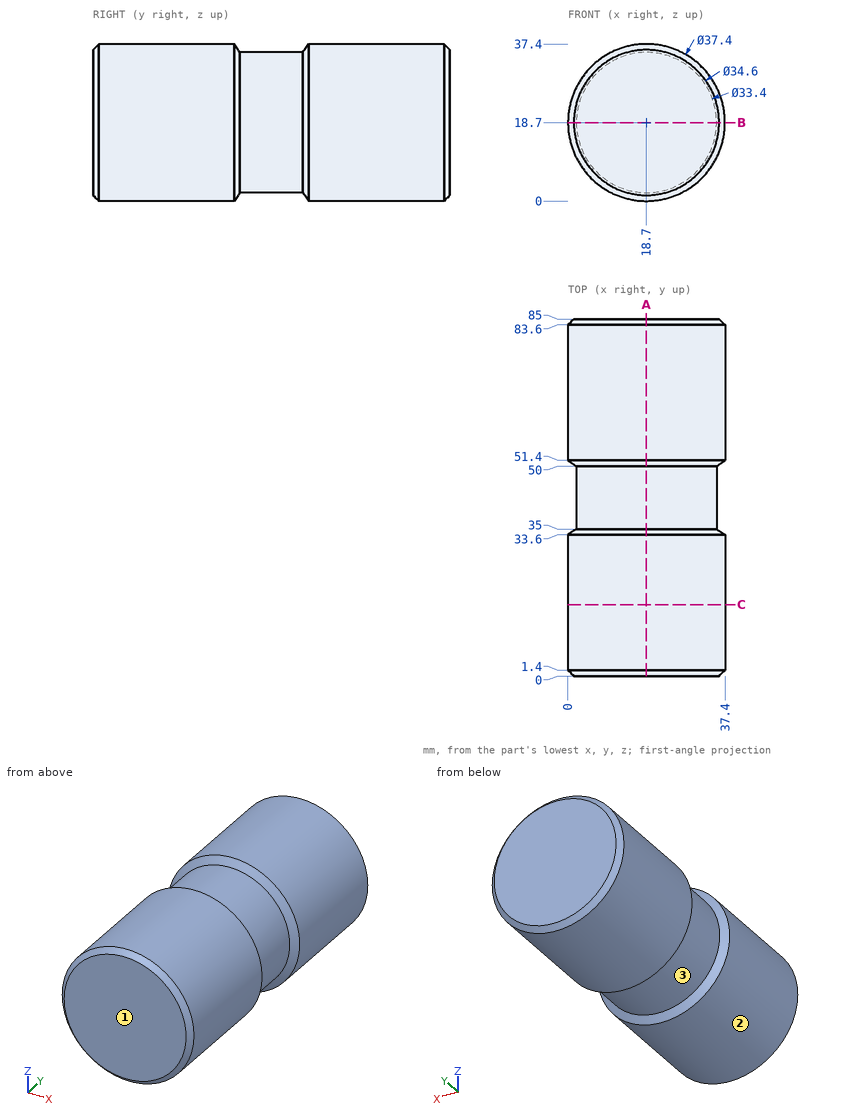
Study the drawing (mm; zero at the part's minimum x, y, z) and answer. Coordinates: 2 decimals unless noted, no trailing zeros. Write each loop counter-clockwise with the first axis right and the second up, starting at its lowest first coordinate (ties: lowest second). Pieces come first, ordered by that corner, then holes. Notation, with made-up numbers: (-21, 32) - (23, 32) arc R12 ccw to (23, 37) - close; hole circle Ø11 at (54.5, -23.5). An arc over 180 degrees is marked (long way). One line per question, with ' | ' between items.
1) Consider probe 1 along Z at (x, y) = (19.5, 78.5); probe 2 along Y at (x, z) = (2, 26) (1 decimal); probe 3 along X at (y, z) = (47.5, 19). Determine where each line is inside the solid, lowest interval first. Write a range as [from, to].
Checks:
probe 1: [0.02, 37.38] | probe 2: [0.9, 33.9], [51.1, 84.1] | probe 3: [2, 35.4]
2) Find section C-C, the plane y = 17. Determine the outline of the cut face in (x, z), and give its area (3 significant figures).
Checks:
outline: circle Ø37.4 at (18.7, 18.7) | area: 1,100 mm2
3) Find section A-A, the plane x = 18.7. Determine the outline of the cut face in (y, z).
Checks:
outline: (0, 1.4) - (1.4, 0) - (33.6, 0) - (35, 2) - (50, 2) - (51.4, 0) - (83.6, 0) - (85, 1.4) - (85, 36) - (83.6, 37.4) - (51.4, 37.4) - (50, 35.4) - (35, 35.4) - (33.6, 37.4) - (1.4, 37.4) - (0, 36) - close
4) Find section B-B, the plane z = 18.7. Determine the outline of the cut face in (x, y).
Checks:
outline: (0, 1.4) - (1.4, 0) - (36, 0) - (37.4, 1.4) - (37.4, 33.6) - (35.4, 35) - (35.4, 50) - (37.4, 51.4) - (37.4, 83.6) - (36, 85) - (1.4, 85) - (0, 83.6) - (0, 51.4) - (2, 50) - (2, 35) - (0, 33.6) - close
5) The mould has two halves that part along Y. Classify the marked faces 1, 2 and 3: +Y half, -Y half, draft (parallel to the pull), parting line (faces both ways), or undercut.
Checks:
face 1: -Y half | face 2: draft | face 3: undercut
6) Flat-ended cylindrical pins translate along their axes: P1, Ø5, axis at y = 27, z = 12.5, coming from the -X side; P2, Ø2, axis at x = 13.5, y = 47, coming from the -Z side. Find the tip coordinate at first contact, or state that the pin passes through.
Checks:
P1: x = 0.37 | P2: z = 2.54
